The listing builds one solid part. Answer for the finished solid, in the listing's coordinates (mm). A direction names the side the tool comes from. Round coordinates to 2 decimals unless told otherwise and drop trailing zeros. Loops run counter-clockwise (first coordinate to the right, second up) from the corner with the lowest first, then second, coordinate; pieces in that order, holes last. Notation, with made-up numbers: (26, 79.5) -> (47, 79.5) arc R8 ccw to (47, 89.5) -> close; hole circle Ø11 at (61.5, 6). An arc over 180 degrees is marked (long way). Use a Markdown table: item, result. Add a question column.
Q1. Section C-C on x = 177 is taken. Give the vertices of the cut face in (y, z).
Q2. Section B-B on z = 0 is taken. Give the vertices of the cut face in (x, y).
Q3. Section A-A on y = -76.2 is taken. Give the vertices of the cut face in (x, z) (3 decimals), then the cut area to 3 significant figures.
Q4. Section D-D on z = 44.5 is taken. Give the vertices of the cut face in (x, y).
Q5. Which of the six approach directions +Z, -Z, +X, -X, +Y, -Y give full straight-line access (tool end or side, diameter ignored) to faces 5 (the flat face through (77, -77, 6.35)), 6 (the flat face through (134, -77, -6.35)), 7 (the flat face through (161.544, -77, 21))?
Q6. Consider line 1 (Z direction, x = 82, y = -64); line 2 (X direction, y = -69, z = 4.5); line 3 (X direction, y = -97.5, z = 10.5). Determine where each line is inside the solid, lowest interval first.
Q7. Given pin 1 Ø1 at (y, z) = (-73.5, 49) entering from +X; pin 2 Ø3 at (x, y) = (166, -69) entering from +Z; pin 3 Ø23 at (y, z) = (-74.5, 26) entering from -X, each flat-ended and moving along its own axis, determine where each tip first touches the part or whether it passes through.
Q8. For a pull along Y with two mould halves and no side action, classify faces 1 (the cylindrical face through (173.574, -73.184, 0.089)), 2 (the flat face through (172, -77, 6.35)), 3 (the flat face through (134, -101.6, 0)), 4 (the cylindrical face through (87.051, -68.513, 0.089)) as released by +Y, released by -Y, zero draft, split by the parting line, or undercut.
from build123d import *

# Parameters (mm, degrees)
F0_R     = 15.875
F1_DEPTH = 50.8
F2_R     = 7.874
F3_DEPTH = 12.7
F5_DEPTH = 76.2
F6_ANGLE = 180


with BuildPart() as f1:
    # F0 (on Front) → F1 (new body)
    with BuildSketch(Plane.XZ):
        Polygon((66.548, -6.35), (66.548, 6.35), (28.448, 6.35), (-28.448, 6.35), (-66.548, 6.35), (-66.548, -6.35), (-28.448, -6.35), (28.448, -6.35), align=None)
        with BuildLine():
            Line((-28.448, 6.35), (28.448, 6.35))
            Line((28.448, 6.35), (28.448, 34.798))
            ThreePointArc((28.448, 34.798), (0, 63.246), (-28.448, 34.798))
            Line((-28.448, 34.798), (-28.448, 6.35))
        make_face()
        with Locations((0, 34.798)):
            Circle(F0_R, mode=Mode.SUBTRACT)
    extrude(amount=F1_DEPTH)

    # F2 (on face) → F3 (cut)
    with BuildSketch(Plane.XY.offset(6.35)):
        with Locations((47.752, -25.4)):
            Circle(F2_R)
        with Locations((-47.752, -25.4)):
            Circle(F2_R)
    extrude(amount=-F3_DEPTH, mode=Mode.SUBTRACT)

    # F4 (on face) → F5 (cut)
    with BuildSketch(Plane(origin=(-28.448, 0, 0), x_dir=(0, -1, 0), z_dir=(-1, 0, 0))):
        Polygon((0, 64.1047875036), (0, 34.798), (9.2448439504, 34.798), (19.9116422636, 64.1047875036), align=None)
        Polygon((0, 34.798), (0, 9.398), (9.2448439504, 34.798), align=None)
    extrude(amount=-F5_DEPTH, mode=Mode.SUBTRACT)


with BuildPart() as f1_1:
    # F6: moved
    add(f1.part.rotate(Axis((66.548, -50.8, 0), (0, 0, -1)), F6_ANGLE))


solid = f1_1.part
Checked values:
| question | item | result |
|---|---|---|
| 1 | outline | (-101.6, -6.35) -> (-83.07, -6.35) -> (-83.07, 6.35) -> (-101.6, 6.35) -> close; (-69.33, -6.35) -> (-50.8, -6.35) -> (-50.8, 6.35) -> (-69.33, 6.35) -> close |
| 2 | outline | (66.55, -101.6) -> (199.64, -101.6) -> (199.64, -50.8) -> (66.55, -50.8) -> close; hole circle Ø15.75 at (85.34, -76.2); hole circle Ø15.75 at (180.85, -76.2) |
| 3 | outline | (66.548, -6.35) -> (77.47, -6.35) -> (77.47, 6.35) -> (66.548, 6.35) -> close; (93.218, -6.35) -> (172.974, -6.35) -> (172.974, 6.35) -> (161.544, 6.35) -> (161.544, 34.798) arc R28.448 ccw to (104.648, 34.798) -> (104.648, 6.35) -> (93.218, 6.35) -> close; (188.722, -6.35) -> (199.644, -6.35) -> (199.644, 6.35) -> (188.722, 6.35) -> close; hole circle Ø31.75 at (133.096, 34.798) |
| 3 | area | 3,390 mm2 |
| 4 | outline | (106.35, -88.82) -> (120.53, -88.82) -> (120.53, -50.8) -> (106.35, -50.8) -> close; (145.66, -88.82) -> (159.84, -88.82) -> (159.84, -50.8) -> (145.66, -50.8) -> close |
| 5 | face 5 | +Z, -X, +Y, -Y |
| 5 | face 6 | -Z, +X, -X, +Y, -Y |
| 5 | face 7 | +Z, +X, +Y, -Y |
| 6 | line 1 | z = -6.35 to 6.35 |
| 6 | line 2 | x = 66.55 to 82.16, 88.53 to 177.66, 184.04 to 199.64 |
| 6 | line 3 | x = 104.65 to 161.54 |
| 7 | pin 1 | stops at x = 158.03 |
| 7 | pin 2 | stops at z = 6.35 |
| 7 | pin 3 | stops at x = 104.65 |
| 8 | face 1 | undercut |
| 8 | face 2 | zero draft |
| 8 | face 3 | released by -Y |
| 8 | face 4 | undercut |
